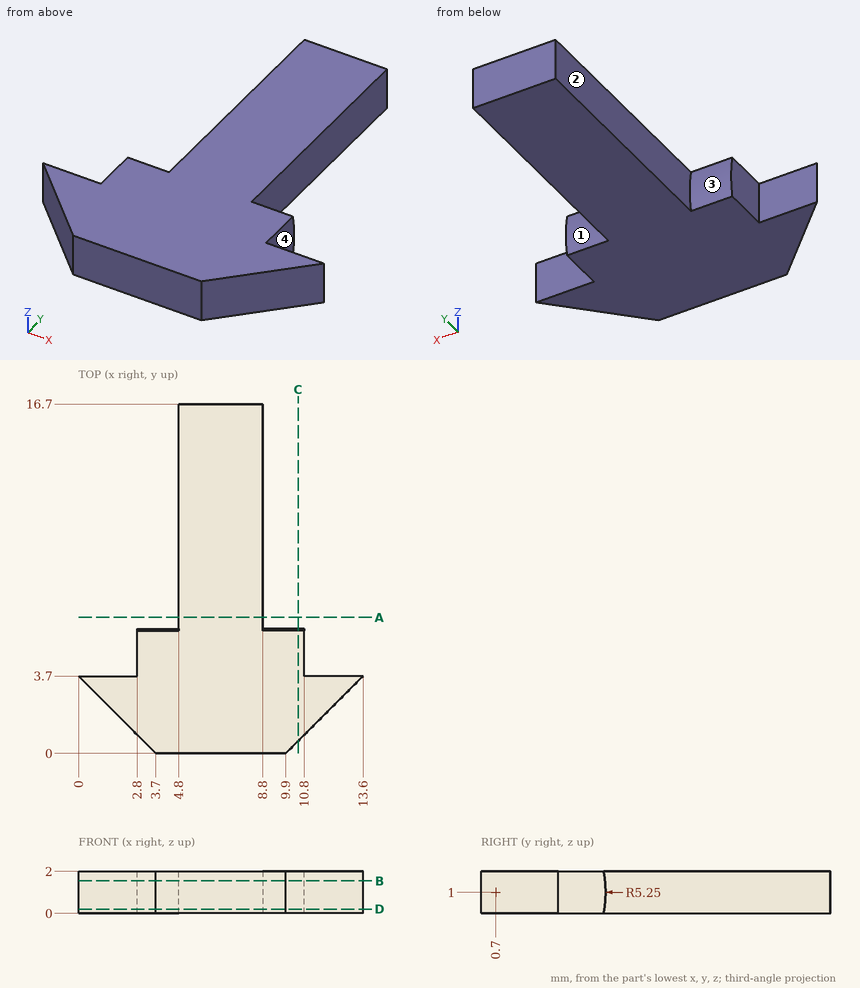
Study the drawing (mm; zero at the part's minimum x, y, z) and answer. A direction names the side the tool comes from. Round coordinates to 2 decimals unless told otherwise and drop trailing zeros. Write each loop counter-clockwise with the first axis right and the second up, starting at its lowest first coordinate (ties: lowest second). Pieces come first, ordered by that corner, then holes.
Q1. Flat-ended cylindrical pins translate along their axes: P1, Ø1, axis at y = 9, z = 1.5, coming from the -X side; P2, Ø1, axis at y = 5, z = 1.5, coming from the -X side; P3, Ø0.6, axis at x = 12.5, z = 1.5, coming from the +Y side. Find the tip coordinate at first contact, or state that the pin passes through.
Values:
P1: stops at x = 4.8
P2: stops at x = 2.8
P3: stops at y = 3.7
Q2. Find section D-D on z = 0.2. Determine the outline of the cut face in (x, y).
Values:
outline: (0, 3.7) - (3.7, 0) - (9.9, 0) - (13.6, 3.7) - (10.8, 3.7) - (10.8, 5.89) - (8.8, 5.89) - (8.8, 16.7) - (4.8, 16.7) - (4.8, 5.89) - (2.8, 5.89) - (2.8, 3.7) - close
Q3. Find section C-C on x = 10.5. Determine the outline of the cut face in (y, z).
Values:
outline: (0.6, 0) - (5.85, 0) arc R5.25 ccw to (5.85, 2) - (0.6, 2) - close
Q4. A tool of negligible diameter and unlimited length cuts with its end or side. For the marked faces 1, 2, 3 and 4, from which of +Z, -Z, +X, -X, +Y, -Y can it reach the whole face along a straight path? Write none if from no direction.
Values:
face 1: +X, +Y
face 2: +Z, -Z, -X, +Y
face 3: -X, +Y
face 4: +Z, -Z, +X, +Y
Q5. Find section B-B on z = 1.55. Determine the outline of the cut face in (x, y), and give its area (3 significant figures).
Values:
outline: (0, 3.7) - (3.7, 0) - (9.9, 0) - (13.6, 3.7) - (10.8, 3.7) - (10.8, 5.92) - (8.8, 5.92) - (8.8, 16.7) - (4.8, 16.7) - (4.8, 5.92) - (2.8, 5.92) - (2.8, 3.7) - close
area: 97.5 mm2
Q6. Straight lines are drawn through the part: line 1 (X direction, y = 5.75, z = 0.85); line 2 (X direction, y = 14, z = 1.05); line 3 (Y direction, x = 12.25, z = 0.3). For each, find the intervals that lie inside material, in ascending order.
Values:
line 1: x = 2.8 to 10.8
line 2: x = 4.8 to 8.8
line 3: y = 2.35 to 3.7
Q7. Find section A-A on y = 6.5. Determine the outline of the cut face in (x, z), and give its area (3 significant figures).
Values:
outline: (4.8, 0) - (8.8, 0) - (8.8, 2) - (4.8, 2) - close
area: 8.00 mm2
